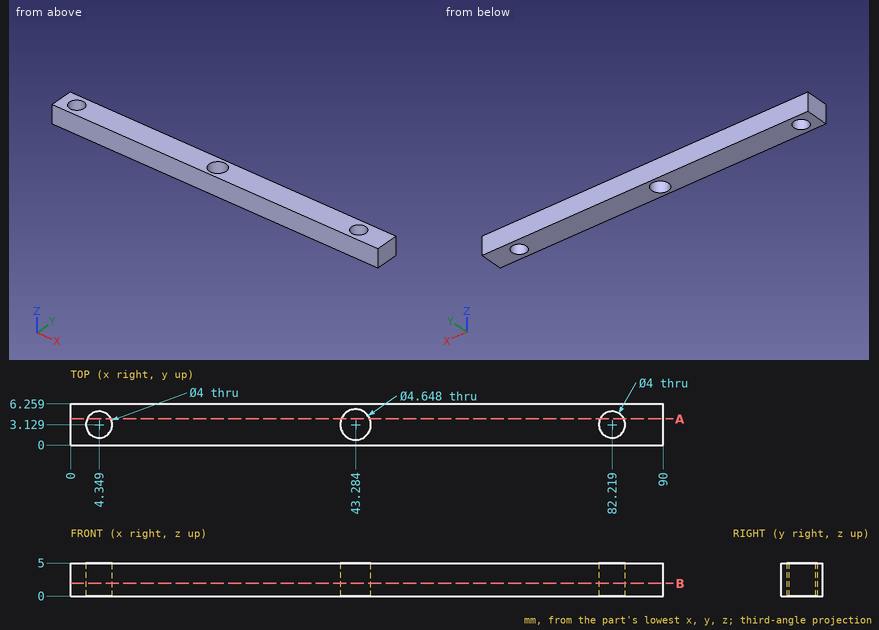
Job drawing, mm, ordinate dimensions from the low corner. One solid piece. Round coordinates to 2 decimals unless told otherwise and drop trailing zeros. Order: outer loops, then holes, each group sorted by start corner. A loop starts at its lowest first (then second) coordinate and runs counter-clockwise, first axis right, second up. Notation, with made-up numbers: (15, -33.5) - (42, -33.5) arc R13 ccw to (42, -29.5) - close; hole circle Ø4 at (22, 53.5). An arc over 180 degrees is marked (long way). Use CSV: the item, a comma, the result in double quotes. Start each with the question number.
1) Saw through at A-A (y = 4). List the corners of the cut face in (x, z).
2) Wall check: L1, parallel to X at y = 3, z = 3.3 (1 decimal); L2, parallel to X at y = 2.25, z = 2.8 (1 decimal); L3, parallel to Y at x = 6, z = 4.6 (1 decimal). Give the ranges that are in metal, low to high. Write a range as [from, to].
3) Saw through at B-B (z = 1.95). List the corners of the cut face in (x, y) (1 decimal).
Values follow:
1,outline,"(0, 0) - (2.55, 0) - (2.55, 5) - (0, 5) - close; (6.15, 0) - (41.13, 0) - (41.13, 5) - (6.15, 5) - close; (45.44, 0) - (80.42, 0) - (80.42, 5) - (45.44, 5) - close; (84.02, 0) - (90, 0) - (90, 5) - (84.02, 5) - close"
2,L1,"x = [0, 2.4], [6.3, 41], [45.6, 80.2], [84.2, 90]"
2,L2,"x = [0, 2.6], [6.1, 41.1], [45.4, 80.4], [84, 90]"
2,L3,"y = [0, 2], [4.3, 6.3]"
3,outline,"(0, 0) - (90, 0) - (90, 6.3) - (0, 6.3) - close; hole circle Ø4 at (4.3, 3.1); hole circle Ø4.6 at (43.3, 3.1); hole circle Ø4 at (82.2, 3.1)"
